Could you check a few things on this model? Use its own coordinates, in mm. Give positions to 0.01 mm unless a question says otherwise; leave off trailing zeros. Write each loop counter-clockwise with the first axis right and the second up, starting at its lowest first coordinate (ties: lowest second). Pieces come first, ordered by that corner, then holes. Notation, with made-up numbers: M 58,12.5 L 76,12.5 A22 ccw 76,47.5 Z; hole C 18.25,-13 d6. An arc over 180 degrees is marked long. Use one line per item in the form item = value.
from build123d import *

# Parameters (mm, degrees)
ESTRUSIONE_ESTRUSIONE1_DEPTH = 6
SMUSSO1_SIZE                 = 0.5


with BuildPart() as part:
    # Schizzo1 → Estrusione-Estrusione1 (new body)
    with BuildSketch(Plane(origin=(0, 0, 0), x_dir=(1, 0, 0), z_dir=(0, 1, 0))):
        with BuildLine():
            Line((-2.5, 4), (2.5, 4))
            ThreePointArc((2.5, 4), (6.5, 0), (2.5, -4))
            Line((2.5, -4), (-2.5, -4))
            ThreePointArc((-2.5, -4), (-6.5, 0), (-2.5, 4))
        make_face()
    extrude(amount=ESTRUSIONE_ESTRUSIONE1_DEPTH)

    # Smusso1
    smusso1_edges = [part.edges().sort_by_distance(p)[0] for p in [
        (6.5, 6, 0),
        (0, 6, -4),
        (-6.5, 6, 0),
        (0, 0, -4),
        (6.5, 0, 0),
        (0, 0, 4),
        (-6.5, 0, 0),
        (0, 6, 4),
    ]]
    chamfer(smusso1_edges, length=SMUSSO1_SIZE)


solid = part.part
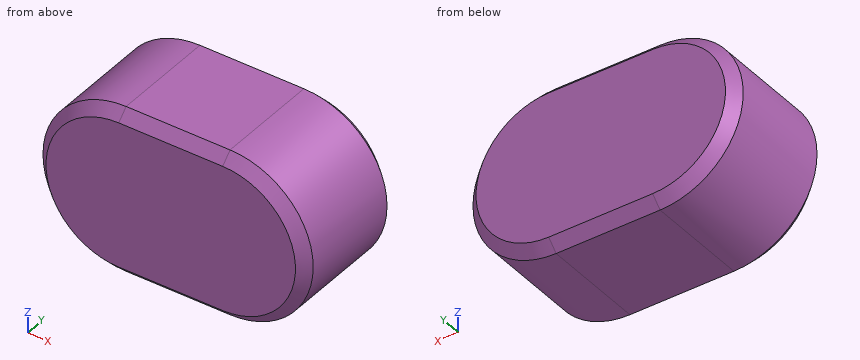
1) I want a section at A-A, the plane y = 1.85. Please give me the cut outline in (x, z).
Checked values:
outline = M -2.5,-4 L 2.5,-4 A4 ccw 2.5,4 L -2.5,4 A4 ccw Z
2) For pin 1 Ø1.5 at (y, z) = (5.5, -2) entering from -X, with a flat end and sliding along its axis, tell me the tip position at first contact or that it passes through.
Checked values:
pin_1 = -6.3
3) If I drill on L1, parallel to X at y = 2.95, z = 0.25; L2, parallel to X at y = 2.3, z = 3.5; L3, parallel to Z at x = -4, y = 3.1, over which ranges is the centre line in solid material (lowest first)?
Checked values:
L1 = -6.49 to 6.49
L2 = -4.44 to 4.44
L3 = -3.71 to 3.71
